Input: part model. Units: mm. Frame: model coordinates. A direction names the side the tool comes from. Round coordinates to 2 decimals unless told otherwise and drop trailing zeros. Order: outer loops, then holes, each group sorted by start corner. A loop starts at its lowest first (then second) coordinate and runs counter-clockwise, first axis right, second up. Notation, with made-up numbers: M -19,20.25 L -13,20.25 A32 cw -13,48.25 Z; hole C 25,23 d9. An arc over 180 degrees is marked long. One line per question, with ' | ' between items.
```python
from build123d import *

# Parameters (mm, degrees)
BOSS_EXTRUDE1_DEPTH = 3
SKETCH1_3_W         = 416
SKETCH1_3_H         = 106
SKETCH1_3_W_2       = 410
SKETCH1_3_H_2       = 100
SKETCH1_3_W_3       = 10
SKETCH1_3_H_3       = 15
SKETCH1_3_H_4       = 10
BOSS_EXTRUDE2_DEPTH = 343
SKETCH2_R           = 5
SKETCH2_W           = 416
SKETCH2_H           = 106
BOSS_EXTRUDE3_DEPTH = 3
SKETCH3_RX          = 1.6
SKETCH3_RY          = 1


with BuildPart() as part:
    # Sketch1 → Boss-Extrude1 (new body)
    with BuildSketch(Plane(origin=(0, 0, 0), x_dir=(1, 0, 0), z_dir=(0, 1, 0))):
        Polygon((-195, 40), (-205, 40), (-205, 35), (-195, 35), (-195, 20), (-205, 10), (-205, -50), (205, -50), (205, 10), (195, 20), (195, 35), (205, 35), (205, 40), (195, 40), (195, 50), (-195, 50), align=None)
    extrude(amount=BOSS_EXTRUDE1_DEPTH)

    # Sketch1_3 → Boss-Extrude2 (add)
    # profile 1 of 7: a face of its own
    with BuildSketch(Plane(origin=(0, 0, 0), x_dir=(1, 0, 0), z_dir=(0, 1, 0))):
        Rectangle(SKETCH1_3_W, SKETCH1_3_H)
        Rectangle(SKETCH1_3_W_2, SKETCH1_3_H_2, mode=Mode.SUBTRACT)
    # profile 2 of 7: a face of its own
    with BuildSketch(Plane(origin=(0, 0, 0), x_dir=(1, 0, 0), z_dir=(0, 1, 0))):
        Polygon((-195, 20), (-205, 20), (-205, 10), align=None)
    # profile 3 of 7: a face of its own
    with BuildSketch(Plane(origin=(0, 0, 0), x_dir=(1, 0, 0), z_dir=(0, 1, 0))):
        with Locations((-200, 27.5)):
            Rectangle(SKETCH1_3_W_3, SKETCH1_3_H_3)
    # profile 4 of 7: a face of its own
    with BuildSketch(Plane(origin=(0, 0, 0), x_dir=(1, 0, 0), z_dir=(0, 1, 0))):
        with Locations((-200, 45)):
            Rectangle(SKETCH1_3_W_3, SKETCH1_3_H_4)
    # profile 5 of 7: a face of its own
    with BuildSketch(Plane(origin=(0, 0, 0), x_dir=(1, 0, 0), z_dir=(0, 1, 0))):
        Polygon((195, 20), (205, 10), (205, 20), align=None)
    # profile 6 of 7: a face of its own
    with BuildSketch(Plane(origin=(0, 0, 0), x_dir=(1, 0, 0), z_dir=(0, 1, 0))):
        with Locations((200, 27.5)):
            Rectangle(SKETCH1_3_W_3, SKETCH1_3_H_3)
    # profile 7 of 7: a face of its own
    with BuildSketch(Plane(origin=(0, 0, 0), x_dir=(1, 0, 0), z_dir=(0, 1, 0))):
        with Locations((200, 45)):
            Rectangle(SKETCH1_3_W_3, SKETCH1_3_H_4)
    extrude(amount=BOSS_EXTRUDE2_DEPTH)

    # Sketch2 → Boss-Extrude3 (add)
    # profile 1 of 3: a face of its own
    with BuildSketch(Plane(origin=(0, 343, 0), x_dir=(1, 0, 0), z_dir=(0, 1, 0))):
        with BuildLine():
            Line((248, -83), (248, 83))
            ThreePointArc((248, 83), (245.071067812, 90.071067812), (238, 93))
            Line((238, 93), (-238, 93))
            ThreePointArc((-238, 93), (-245.071067812, 90.071067812), (-248, 83))
            Line((-248, 83), (-248, -83))
            ThreePointArc((-248, -83), (-245.071067812, -90.071067812), (-238, -93))
            Line((-238, -93), (238, -93))
            ThreePointArc((238, -93), (245.071067812, -90.071067812), (248, -83))
        make_face()
        with Locations(Location((-233, 38, 0), (0, 0, 270))):
            Circle(SKETCH2_R, mode=Mode.SUBTRACT)
        with Locations(Location((-233, -38, 0), (0, 0, 270))):
            Circle(SKETCH2_R, mode=Mode.SUBTRACT)
        with Locations(Location((-193, -78, 0), (0, 0, 270))):
            Circle(SKETCH2_R, mode=Mode.SUBTRACT)
        with Locations(Location((-193, 78, 0), (0, 0, 270))):
            Circle(SKETCH2_R, mode=Mode.SUBTRACT)
        with Locations(Location((193, 78, 0), (0, 0, 270))):
            Circle(SKETCH2_R, mode=Mode.SUBTRACT)
        with Locations(Location((233, 38, 0), (0, 0, 270))):
            Circle(SKETCH2_R, mode=Mode.SUBTRACT)
        with Locations(Location((233, -38, 0), (0, 0, 270))):
            Circle(SKETCH2_R, mode=Mode.SUBTRACT)
        with Locations(Location((193, -78, 0), (0, 0, 270))):
            Circle(SKETCH2_R, mode=Mode.SUBTRACT)
        with Locations(Location((93, -78, 0), (0, 0, 270))):
            Circle(SKETCH2_R, mode=Mode.SUBTRACT)
        with Locations(Location((-93, -78, 0), (0, 0, 270))):
            Circle(SKETCH2_R, mode=Mode.SUBTRACT)
        with Locations(Location((-93, 78, 0), (0, 0, 270))):
            Circle(SKETCH2_R, mode=Mode.SUBTRACT)
        with Locations(Location((93, 78, 0), (0, 0, 270))):
            Circle(SKETCH2_R, mode=Mode.SUBTRACT)
        with Locations(Location((0, 78, 0), (0, 0, 270))):
            Circle(SKETCH2_R, mode=Mode.SUBTRACT)
        with Locations(Location((0, -78, 0), (0, 0, 270))):
            Circle(SKETCH2_R, mode=Mode.SUBTRACT)
        with BuildLine():
            Line((-218, 53), (-218, -53))
            ThreePointArc((-218, -53), (-215.071067812, -60.071067812), (-208, -63))
            Line((-208, -63), (208, -63))
            ThreePointArc((208, -63), (215.071067812, -60.071067812), (218, -53))
            Line((218, -53), (218, 53))
            ThreePointArc((218, 53), (215.071067812, 60.071067812), (208, 63))
            Line((208, 63), (-208, 63))
            ThreePointArc((-208, 63), (-215.071067812, 60.071067812), (-218, 53))
        make_face(mode=Mode.SUBTRACT)
    # profile 2 of 3: a face of its own
    with BuildSketch(Plane(origin=(0, 343, 0), x_dir=(1, 0, 0), z_dir=(0, 1, 0))):
        with BuildLine():
            ThreePointArc((-218, 53), (-215.071067812, 60.071067812), (-208, 63))
            Line((-208, 63), (208, 63))
            ThreePointArc((208, 63), (215.071067812, 60.071067812), (218, 53))
            Line((218, 53), (218, -53))
            ThreePointArc((218, -53), (215.071067812, -60.071067812), (208, -63))
            Line((208, -63), (-208, -63))
            ThreePointArc((-208, -63), (-215.071067812, -60.071067812), (-218, -53))
            Line((-218, -53), (-218, 53))
        make_face()
        Rectangle(SKETCH2_W, SKETCH2_H, mode=Mode.SUBTRACT)
    # profile 3 of 3: a face of its own
    with BuildSketch(Plane(origin=(0, 343, 0), x_dir=(1, 0, 0), z_dir=(0, 1, 0))):
        Rectangle(SKETCH2_W, SKETCH2_H)
        Polygon((-205, 40), (-195, 40), (-195, 50), (195, 50), (195, 40), (205, 40), (205, 35), (195, 35), (195, 20), (205, 10), (205, -50), (-205, -50), (-205, 10), (-195, 20), (-195, 35), (-205, 35), align=None, mode=Mode.SUBTRACT)
    extrude(amount=BOSS_EXTRUDE3_DEPTH)

    # Cut-Sweep2: sweep along a path in Sketch4
    with BuildLine(Plane(origin=(0, 346, 0), x_dir=(1, 0, 0), z_dir=(0, 1, 0))) as cut_sweep2_path:
        Line((-208, 63), (208, 63))
        ThreePointArc((208, 63), (215.071067812, 60.071067812), (218, 53))
        Line((218, 53), (218, -53))
        ThreePointArc((218, -53), (215.071067812, -60.071067812), (208, -63))
        Line((208, -63), (-208, -63))
        ThreePointArc((-208, -63), (-215.071067812, -60.071067812), (-218, -53))
        Line((-218, -53), (-218, 53))
        ThreePointArc((-218, 53), (-215.071067812, 60.071067812), (-208, 63))
    # Sketch3 → Cut-Sweep2 (sweep, cut)
    with BuildSketch(Plane.XY):
        with Locations((-218, 346)):
            Ellipse(SKETCH3_RX, SKETCH3_RY)
    sweep(path=cut_sweep2_path.line, mode=Mode.SUBTRACT)


solid = part.part
```
Item 1: Line query: line 1 along X through (y, z) = (344.5, 78); line 2 along X through (y, z) = (343.75, -38); line 3 along Z through (x, y) = (166, 282). Output: solid intervals per line, ascending. Write a range as from..to.
Report:
line 1: -248..-198, -188..-98, -88..-5, 5..88, 98..188, 198..248 | line 2: -248..-238, -228..-205, 205..228, 238..248 | line 3: -53..-50, 50..53
Item 2: First-contact query: pin 1 (6 mm diameter, centred on y = 87.5, z = -20.5, fed in from +X); pin 2 (11.5 mm diameter, centred on x = -233, z = 38, fed in from -Y); pin 3 (5 mm diameter, centred on x = 201, y = 91, fed in from +Z). Flat tips, straight axial feed; report the tip coordinate or a pass-through.
Report:
pin 1: x = 208 | pin 2: y = 343 | pin 3: z = 53
Item 3: Mould query, pull axis Z, two halves, no side actions, for faces 4 (the cylindrical face through (-245.15, 344.48, 89.99)), 5 (the cylindrical face through (197, 344, -75)), 6 (the flat face through (-3, 0, -1)). Classes: +Z half, -Z half, draft (parallel to the pull), parting line (faces both ways), or undercut.
Report:
face 4: +Z half | face 5: undercut | face 6: draft
Item 4: Access query for faces 1 (the flat face through (-195, 172, -45)), 2 (the flat face through (-3, 169, 53)), 3 (the flat face through (208, 169, 1)). Directions: +Z, -Z, +X, -X, +Y, -Y. A direction counts if a zero-diameter tool reaches every point of the face in a straight line with its end or side. Return the directions, or none.
Report:
face 1: +Y | face 2: +Z, +X, -X, -Y | face 3: +Z, -Z, +X, -Y
Item 5: Section query A-A, the plane y = 142. Return loops of the section in (x, z), plus the area to 3 significant figures.
Report:
outline: M -208,-53 L 208,-53 L 208,53 L -208,53 Z; hole M -205,-40 L -195,-40 L -195,-50 L 195,-50 L 195,-40 L 205,-40 L 205,-35 L 195,-35 L 195,-20 L 205,-10 L 205,50 L -205,50 L -205,-10 L -195,-20 L -195,-35 L -205,-35 Z | area: 3,700 mm²
